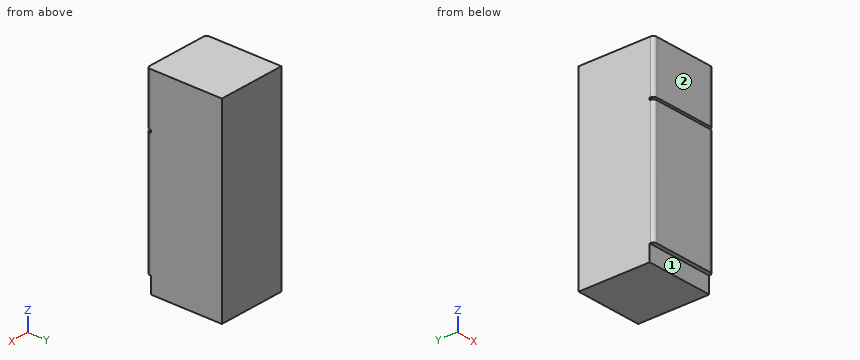
from build123d import *

# Parameters (mm, degrees)
F1_W     = 590
F1_H     = 650
F2_DEPTH = 1670
F3_W     = 35
F3_H     = 140
F3_H_2   = 20
F4_DEPTH = 590.001
F5_R     = 30


with BuildPart() as f2:
    # F1 (on Top) → F2 (new body)
    with BuildSketch(Plane.XY):
        with Locations((295, 325)):
            Rectangle(F1_W, F1_H)
    extrude(amount=F2_DEPTH)

    # F3 (on face) → F4 (cut, through all)
    with BuildSketch(Plane.YZ.offset(590)):
        with Locations((17.5, 70)):
            Rectangle(F3_W, F3_H)
        with Locations((17.5, 1210)):
            Rectangle(F3_W, F3_H_2)
    extrude(amount=-F4_DEPTH, mode=Mode.SUBTRACT)

    # F5
    f5_edges = [f2.edges().sort_by_distance(p)[0] for p in [
        (0, 0, 1445),
        (0, 0, 670),
        (590, 0, 670),
        (590, 0, 1445),
    ]]
    fillet(f5_edges, radius=F5_R)


solid = f2.part
Read the model definition and answer for the solid it produces. Units are mm, in the model's axes. Face numbers are marked on the shaded views. A direction names the side the tool comes from. Give positions to 0.01 mm unless a question says otherwise; leave off trailing zeros. Answer in a Markdown table with one row per item. Add a question column.
Item 1: A tool of negligible diameter and unlimited length cuts with its end or side. For the marked faces 1 and 2, from which of +Z, -Z, +X, -X, +Y, -Y can it reach the whole face along a straight path? Write none if from no direction.
Item 2: Flat-ended cylindrical pins translate along their axes: P1, Ø10.5, axis at x = 357.5, y = 15.5, coming from the -Z side; P2, Ø6, axis at x = 343, z = 1212, coming from the -Y side. Find the tip coordinate at first contact, or state that the pin passes through.
Item 3: Find the intervals of material crossed by L1, parallel to Y at x = 121, z = 69, in increasing order.
Recorded:
| question | item | result |
|---|---|---|
| 1 | face 1 | -Z, +X, -X, -Y |
| 1 | face 2 | +Z, -Z, +X, -X, -Y |
| 2 | P1 | stops at z = 140 |
| 2 | P2 | stops at y = 35 |
| 3 | L1 | y = 35 to 650 |
